Design review of the part shown in the three views and the two pictorial views. Dimensions are in mm from the part's minimum x, y and z. A direction names the side the tool comes from. Round coordinates to 2 decimals unless told otherwise and drop trailing zeros. Write each loop counter-clockwise with the first axis right and the second up, starting at its lowest first coordinate (ties: lowest second). Pieces come first, ordered by that corner, then holes. Notation, with made-up numbers: (11, 9.5) -> (26, 9.5) arc R26 cw to (26, 39.5) -> close; hole circle Ø7 at (-39.5, 1.5). An arc over 180 degrees is marked (long way). One line per question, with ' | ' between items. Start each with the question number.
1) For the marked faces 4, 5, 6, 7 and 8, list the 3-axis set-ups (+Z, -Z, +X, -X, +Y, -Y) from which the entire face can be reached by the end or side of a thin tool; tool diameter is ignored.
2) Insertion check: pin 1 Ø6 at (x, y) = (81.5, 9) entering from +Z; pin 2 Ø5 at (x, y) = (100.5, 22) entering from +Z; pin 3 Ø6 at (x, z) = (99.5, 22.5) entering from -Y. Each pin has a flat end and moves straight along its axis. Give the tip position at first contact, or say it passes through.
3) Consider section C-C (x = 117). Count the separate pieces of the cut face and the enclosed holes in it, then the cut area to 3 significant figures.
4) Consider section B-B (y = 37.5). Give the boundary of the cut face in (x, z), then the cut area to 3 significant figures.
5) Consider section D-D (y = 49). Give the boundary of the cut face in (x, z), then the cut area to 3 significant figures.
6) Consider section A-A (z = 80.5). Give the boundary of the cut face in (x, y).
7) For probe 1 along X at (y, z) = (31, 74.5); probe 2 along Y at (x, z) = (15.5, 36); probe 3 along Y at (x, z) = (114, 36.5), list the stretches that pass through material, from the lowest coordinate up.
8) Mouldability with a two-part tool opening along X and no side actions: class the marked faces 1, 2 and 3 as +X half, -X half, draft (parallel to the pull), parting line (faces both ways), or undercut.
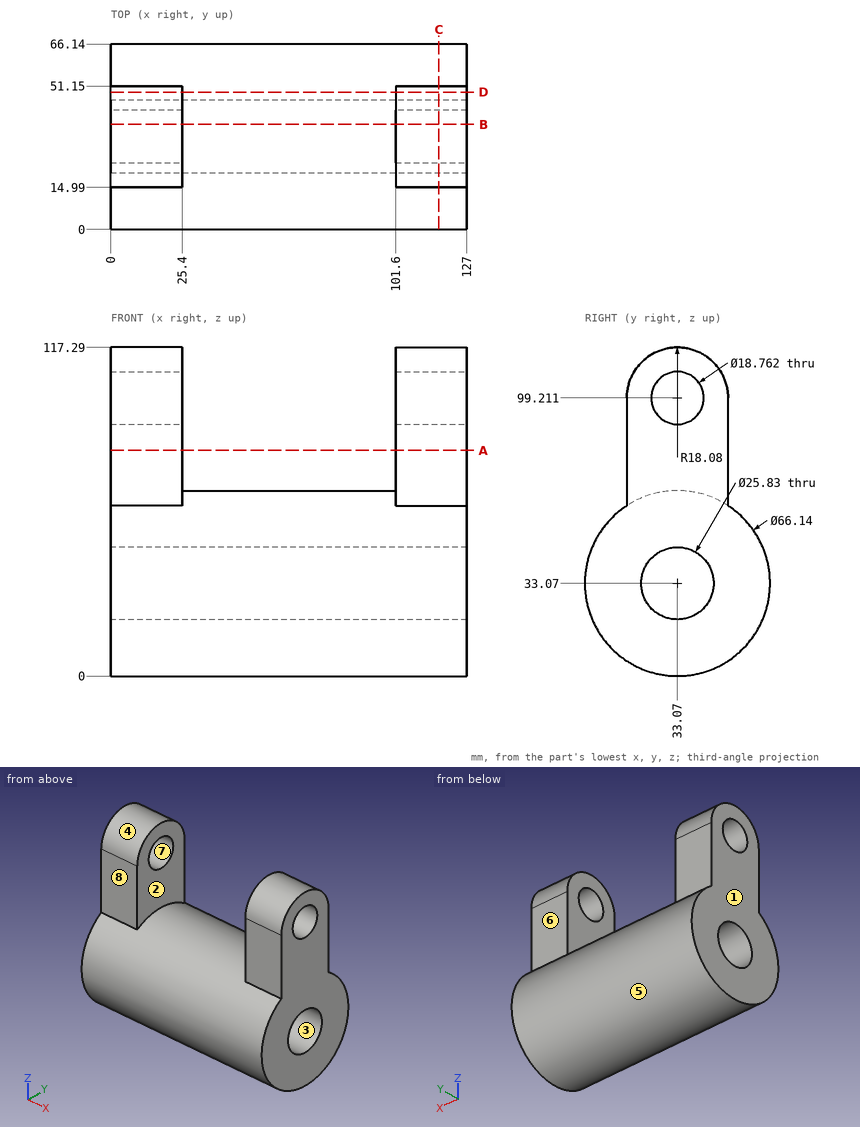
From the geometry:
1) face 4: +Z, +X, -X | face 5: none | face 6: +Z, +X, -X, +Y | face 7: +X, -X | face 8: +Z, +X, -X, -Y
2) pin 1: stops at z = 58.56 | pin 2: stops at z = 114.99 | pin 3: stops at y = 0.88
3) separate pieces: 1 | enclosed holes: 2 | area: 4,410 mm2
4) outline: (0, 0.3) -> (127, 0.3) -> (127, 20.94) -> (0, 20.94) -> close; (0, 45.2) -> (127, 45.2) -> (127, 90.94) -> (101.6, 90.94) -> (101.6, 65.84) -> (25.4, 65.84) -> (25.4, 90.94) -> (0, 90.94) -> close; (0, 107.48) -> (25.4, 107.48) -> (25.4, 116.74) -> (0, 116.74) -> close; (101.6, 107.48) -> (127, 107.48) -> (127, 116.74) -> (101.6, 116.74) -> close | area: 6,990 mm2
5) outline: (0, 4.09) -> (127, 4.09) -> (127, 107.76) -> (101.6, 107.76) -> (101.6, 62.05) -> (25.4, 62.05) -> (25.4, 107.76) -> (0, 107.76) -> close | area: 9,680 mm2
6) outline: (0, 14.99) -> (25.4, 14.99) -> (25.4, 51.15) -> (0, 51.15) -> close; (101.6, 14.99) -> (127, 14.99) -> (127, 51.15) -> (101.6, 51.15) -> close
7) probe 1: x = 0 to 25.4, 101.6 to 127 | probe 2: y = 0.13 to 20.49, 45.65 to 66.01 | probe 3: y = 0.18 to 20.62, 45.52 to 65.96
8) face 1: -X half | face 2: undercut | face 3: draft
